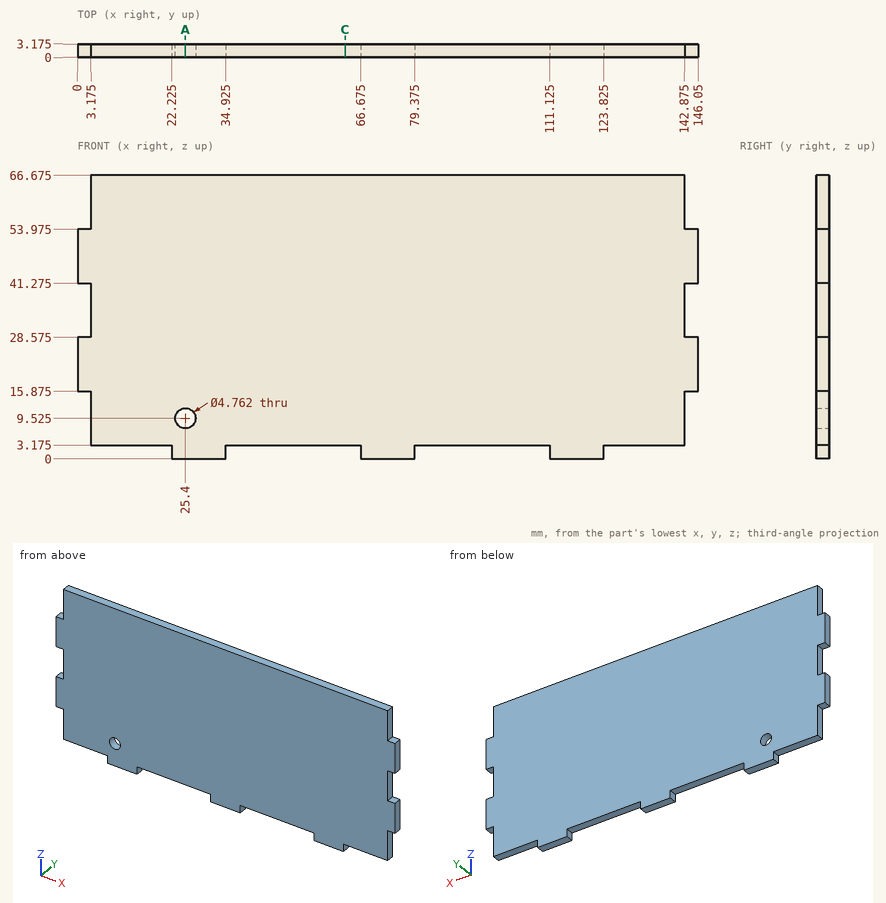
Source: three-view drawing plus pictorial views. Frame: mm from the lowest corner of the part. Round coordinates to 2 decimals unless told otherwise and drop trailing zeros. Loops run counter-clockwise (first coordinate to the right, second up) from the corner with the lowest first, then second, coordinate; pieces in that order, holes last. Notation, with made-up numbers: (89, -23.5) -> (97, -23.5) arc R35 ccw to (97, 12.5) -> close; hole circle Ø4 at (72, 51.25). An arc over 180 degrees is marked (long way). Use one line per item in the form item = value.
Item 1: Cut plane C-C on x = 63. Output: boundary loops of the cut face in (y, z) (1 decimal).
Evaluation:
outline = (0, 3.2) -> (3.2, 3.2) -> (3.2, 66.7) -> (0, 66.7) -> close
Item 2: Material intervals for probe 1 along X at (y, z) = (0.65, 3) (1 decimal); probe 2 along Z at (x, y) = (25.4, 2.15) (1 decimal); probe 3 along X at (y, z) = (0.85, 55) (1 decimal), sorted ascending.
Evaluation:
probe_1 = 22.2 to 34.9, 66.7 to 79.4, 111.1 to 123.8
probe_2 = 0 to 7.1, 11.9 to 66.7
probe_3 = 3.2 to 142.9
Item 3: Cut plane A-A on x = 25.4. Output: boundary loops of the cut face in (y, z) (1 decimal).
Evaluation:
outline = (0, 0) -> (3.2, 0) -> (3.2, 7.1) -> (0, 7.1) -> close; (0, 11.9) -> (3.2, 11.9) -> (3.2, 66.7) -> (0, 66.7) -> close
Item 4: Contact query for flat-ended pins moving along their axis: pin 1 Ø3 at (x, z) = (25.4, 9.525) entering from +Y; pin 2 Ø1.6 at (x, y) = (144.5, 1) entering from -Z (1 decimal); pin 3 Ø1 at (x, y) = (53, 1.5) entering from -Z (1 decimal); pin 4 Ø1.6 at (x, y) = (2, 1) entering from +Z (1 decimal). Output: stop coordinate, or through.
Evaluation:
pin_1 = through
pin_2 = 15.9
pin_3 = 3.2
pin_4 = 54
